```python
from build123d import *

# Parameters (mm, degrees)
SKETCH005_R          = 35
SKETCH005_R_2        = 25
PAD_DEPTH            = 10
SKETCH006_R          = 32.2
SKETCH006_R_2        = 25
PAD001_DEPTH         = 3
SKETCH_R             = 35
SKETCH_R_2           = 28
PAD002_DEPTH         = 17
SKETCH004_R          = 1.5
POCKET_DEPTH         = 20
SKETCH003_R          = 1.5
POCKET001_DEPTH      = 8.5
POCKET001_DEPTH_BACK = 100
PAD003_DEPTH         = 0.01
PAD003_DEPTH_BACK    = 17
POLARPATTERN_COUNT   = 4


with BuildPart() as part:
    # Sketch005 → Pad (new body)
    with BuildSketch(Plane.XY.offset(-1.5)):
        Circle(SKETCH005_R)
        Circle(SKETCH005_R_2, mode=Mode.SUBTRACT)
    extrude(amount=-PAD_DEPTH)

    # Sketch006 → Pad001 (join)
    with BuildSketch(Plane.XY.offset(-1.5)):
        Circle(SKETCH006_R)
        Circle(SKETCH006_R_2, mode=Mode.SUBTRACT)
    extrude(amount=PAD001_DEPTH)

    # Sketch → Pad002 (join)
    with BuildSketch(Plane.XY.offset(1.5)):
        Circle(SKETCH_R)
        Circle(SKETCH_R_2, mode=Mode.SUBTRACT)
    extrude(amount=PAD002_DEPTH)

    # Sketch004 → Pocket (cut)
    with BuildSketch(Plane(origin=(28, 0, 0), x_dir=(1, 0, 0), z_dir=(0, 0, 1))):
        Circle(SKETCH004_R)
    extrude(amount=POCKET_DEPTH, mode=Mode.SUBTRACT)

    # Sketch003 → Pocket001 (cut, two sides)
    with BuildSketch(Plane(origin=(35, 0, 0), x_dir=(0, 0.939693, 0.34202), z_dir=(1, 0, 0))) as pocket001_sk:
        Circle(SKETCH003_R)
    extrude(amount=-POCKET001_DEPTH, mode=Mode.SUBTRACT)
    extrude(pocket001_sk.sketch, amount=POCKET001_DEPTH_BACK, mode=Mode.SUBTRACT)

    # Sketch002 → Pad003 (join, two sides)
    with BuildSketch(Plane.XY.offset(-1.5)) as pad003_sk:
        with BuildLine():
            ThreePointArc((-34.997021, 0.456663), (-33.922719, -8.616793), (-30.53664, -17.103029))
            Line((-30.53664, -17.103029), (-21.762611, -12.504957))
            ThreePointArc((-25.093421, 0), (-24.251171, -6.471733), (-21.762611, -12.504957))
            Line((-34.997021, 0.456663), (-25.093421, 0))
        make_face()
    pad003 = extrude(amount=PAD003_DEPTH) + extrude(pad003_sk.sketch, amount=-PAD003_DEPTH_BACK)

    # PolarPattern: Pad003 ×4 about axis
    polarpattern_axis = Axis((0, 0, -1.5), (0, 0, 1))
    for i in range(1, POLARPATTERN_COUNT):
        add(pad003.rotate(polarpattern_axis, i * 360 / POLARPATTERN_COUNT))


solid = part.part
```
The model under review builds one solid part; all positions refer to its coordinate system, in mm. A direction names the side the tool comes from. Round coordinates to 2 decimals unless told otherwise and drop trailing zeros. Loops run counter-clockwise (first coordinate to the right, second up) from the corner with the lowest first, then second, coordinate; pieces in that order, holes last. Notation, with made-up numbers: (-10.75, 83) - (45.25, 83) arc R19 cw to (45.25, 109) - close; hole circle Ø3 at (84, -35.75). An arc over 180 degrees is marked (long way). Use a Markdown table: item, result. Add a question column.
Q1. Insertion check: pin 1 Ø1.5 at (x, z) = (0.5, 12.5) entering from -Y; pin 2 Ø1 at (x, z) = (-15.5, 4.5) entering from -Y; pin 3 Ø8 at (y, z) = (20, -14.5) entering from -X. Each pin has a flat end and moves straight along its axis. Give the tip position at first contact, or say it passes through.
Q2. The part is to be moulded in two halves that separate along X. For faces 1 (the face through (-17, 19, 1.5)), 2 (the face through (14.836, -26.211, -15.049)), 3 (the face through (28.2, -16.5, -1.5)), say which applies: pulls with the +X half, pulls with the -X half, needs draft (parallel to the pull), parting line crosses it, or undercut.
Q3. Add section A-A (x = -9). State the section outline as (y, z) points, plus the area to 3 significant figures.
Q4. Add section D-D (y = -11.5). State the section outline as (x, z) points, plus the area to 3 significant figures.
Q5. Machinability: for faces 4 (the face through (16.5, 28.3, -1.5)), 5 (the face through (30.713, 9.672, -0.021)), 6 (the face through (8, -32, -1.49)), 7 (the face through (-26.211, -14.836, -14.951)), which of the approach directions +Z, -Z, +X, -X, +Y, -Y give a long, thin tool a straight path to every point of the face, cutting with its end or side? Answer none if there is none.
Q6. For probe 1 along Y at (x, z) = (0, 6.25); probe 2 along Y at (x, z) = (1, -11); probe 3 along Z at (x, y) = (25, 5), list the stretches that pass through material, from the lowest coordinate up.
Q7. Add section C-C (z = -10.5). State the section outline as (x, y) points, plus the area to 3 significant figures.
Worked answers:
| question | item | result |
|---|---|---|
| 1 | pin 1 | y = -35 |
| 1 | pin 2 | y = -31.62 |
| 1 | pin 3 | x = -30.39 |
| 2 | face 1 | undercut |
| 2 | face 2 | pulls with the +X half |
| 2 | face 3 | needs draft |
| 3 | outline | (-33.82, -11.5) - (-23.32, -11.5) - (-23.32, 1.5) - (-26.51, 1.5) - (-26.51, 18.5) - (-33.82, 18.5) - (-33.82, 1.5) - (-30.92, 1.5) - (-30.92, -1.5) - (-33.82, -1.5) - close; (23.32, -11.5) - (23.43, -11.5) - (23.43, -18.5) - (33.82, -18.5) - (33.82, -1.49) - (30.92, -1.49) - (30.92, 1.5) - (33.82, 1.5) - (33.82, 18.5) - (26.51, 18.5) - (26.51, 1.5) - (23.32, 1.5) - close |
| 3 | area | 577 mm² |
| 4 | outline | (-33.06, -18.5) - (-22.31, -18.5) - (-22.31, -11.5) - (-22.2, -11.5) - (-22.2, 1.5) - (-25.53, 1.5) - (-25.53, 18.5) - (-33.06, 18.5) - (-33.06, 1.5) - (-30.08, 1.5) - (-30.08, -1.49) - (-33.06, -1.49) - close; (22.2, -11.5) - (33.06, -11.5) - (33.06, -1.5) - (30.08, -1.5) - (30.08, 1.5) - (33.06, 1.5) - (33.06, 18.5) - (25.53, 18.5) - (25.53, 1.5) - (22.2, 1.5) - close |
| 4 | area | 596 mm² |
| 5 | face 4 | +X, +Y |
| 5 | face 5 | none |
| 5 | face 6 | +X, -Y |
| 5 | face 7 | -Z, +X, -Y |
| 6 | probe 1 | -35 to -28, 28 to 35 |
| 6 | probe 2 | -34.99 to -24.98, 24.98 to 34.99 |
| 6 | probe 3 | -18.5 to 1.5 |
| 7 | outline | circle Ø70 at (0, 0); hole circle Ø50 at (0, 0) |
| 7 | area | 1,880 mm² |
